Part print with two shaded views. Sizes in mm from the minimum x, y, z corner. Coordinates: 2 decimals unless noted, no trailing zeros. Order: outer loops, then holes, each group sorted by start corner. A loop starts at its lowest first (then second) coordinate and runs counter-clockwise, first axis right, second up. Notation, with made-up numbers: M 64,11 L 115,11 A21 ccw 115,44 Z; hole C 27,19.5 d3. An arc over 180 degrees is marked long. Answer in a Markdown table with one row per item. Add a question column.
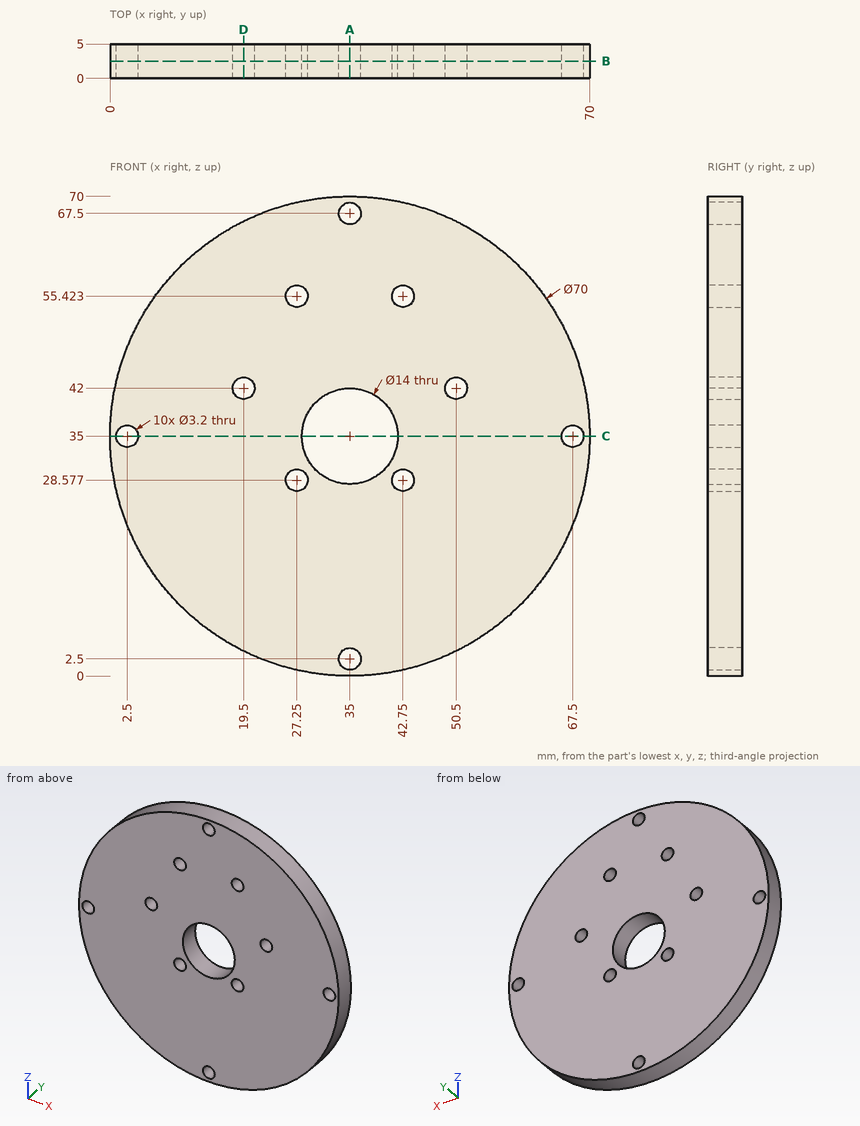
(1) Slice it at C-C (z = 35). List the corners of the cut face in (x, y).
(2) Slice it at D-D (x = 19.5). List the corners of the cut face in (y, z), and give its area (3 significant figures).
(3) Wall check: line 1 (Z direction, x = 67.5, y = 3.1) (1 decimal); line 2 (X direction, y = 1.75, z = 31) (1 decimal); line 3 (Z direction, x = 40, y = 1.95). Give the ranges that are in metal, low to high.
(4) Drop flat-ended pins along their axis: P1, Ø1.9, axis at x = 67.5, z = 35, coming from the +Y side; P2, Ø2, axis at y = 1, z = 15.5, coming from the +X side; P3, Ø3, axis at x = 44.5, y = 3.5, coming from the -Z side; P4, Ø1, axis at x = 47, y = 4, coming from the -Z side. Give the stop position or say it passes through.
(5) Slice it at A-A (x = 35). List the corners of the cut face in (y, z), and give its area (3 significant figures).
(6) Slice it at B-B (y = 2.5). State how many separate pieces and enclosed holes the cut face has, and give its area (3 significant figures).
Computed:
| question | item | result |
|---|---|---|
| 1 | outline | M 0,0 L 0.9,0 L 0.9,5 L 0,5 Z; M 4.1,0 L 28,0 L 28,5 L 4.1,5 Z; M 42,0 L 65.9,0 L 65.9,5 L 42,5 Z; M 69.1,0 L 70,0 L 70,5 L 69.1,5 Z |
| 2 | outline | M 0,3.62 L 5,3.62 L 5,40.4 L 0,40.4 Z; M 0,43.6 L 5,43.6 L 5,66.38 L 0,66.38 Z |
| 2 | area | 298 mm^2 |
| 3 | line 1 | z = 22 to 33.4, 36.6 to 48 |
| 3 | line 2 | x = 0.2 to 29.3, 40.7 to 69.8 |
| 3 | line 3 | z = 0.36 to 30.1, 39.9 to 69.64 |
| 4 | P1 | passes through |
| 4 | P2 | stops at x = 64.71 |
| 4 | P3 | stops at z = 0.93 |
| 4 | P4 | stops at z = 1.94 |
| 5 | outline | M 0,0 L 5,0 L 5,0.9 L 0,0.9 Z; M 0,4.1 L 5,4.1 L 5,28 L 0,28 Z; M 0,42 L 5,42 L 5,65.9 L 0,65.9 Z; M 0,69.1 L 5,69.1 L 5,70 L 0,70 Z |
| 5 | area | 248 mm^2 |
| 6 | separate pieces | 1 |
| 6 | enclosed holes | 11 |
| 6 | area | 3,610 mm^2 |
